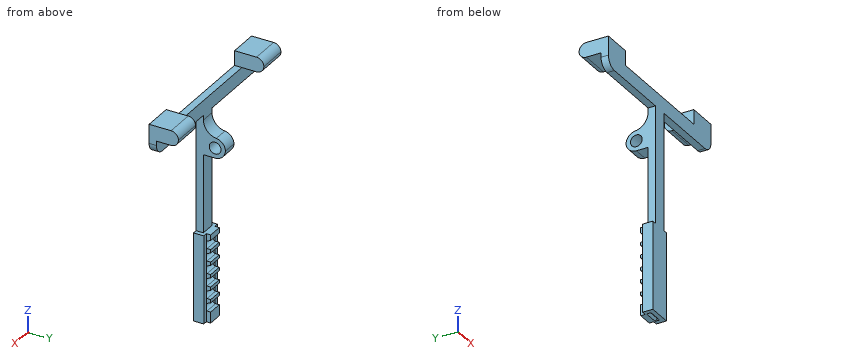
from build123d import *

# Parameters (mm, degrees)
BOSS_EXTRUDE1_DEPTH = 5
SKETCH1_3_W         = 20
SKETCH1_3_H         = 10
SKETCH1_3_W_2       = 10
SKETCH1_3_H_2       = 13.608990902
BOSS_EXTRUDE2_DEPTH = 20
SKETCH1_5_W         = 10
SKETCH1_5_H         = 60
BOSS_EXTRUDE3_DEPTH = 10
SKETCH3_R           = 4
CUT_EXTRUDE1_DEPTH  = 10
FILLET1_R           = 10
FILLET2_R           = 5
FILLET3_R           = 7
FILLET4_R           = 7
FILLET5_R           = 7
SKETCH1_6_W         = 3
SKETCH1_6_H         = 60
BOSS_EXTRUDE4_DEPTH = 7


# Some blends are built 0.0001 mm under size
with BuildPart() as part:
    # Sketch1 → Boss-Extrude1 (new body)
    with BuildSketch(Plane(origin=(0, 0, 0), x_dir=(1, 0, 0), z_dir=(0, 1, 0))):
        Polygon((40, -8.515763432), (40, -18.515763432), (60, -18.515763432), (60, 1.484236568), (5, 1.484236568), (5, 141.484236568), (-5, 141.484236568), (-5, 1.484236568), (-60, 1.484236568), (-60, -18.515763432), (-40, -18.515763432), (-40, -8.515763432), align=None)
    extrude(amount=BOSS_EXTRUDE1_DEPTH)

    # Sketch1<3> → Boss-Extrude2 (add)
    with BuildSketch(Plane(origin=(0, 0, 0), x_dir=(1, 0, 0), z_dir=(0, 1, 0))):
        with Locations((-50, -13.515763432)):
            Rectangle(SKETCH1_3_W, SKETCH1_3_H)
        Polygon((60, -8.515763432), (44.667493795, -8.515763432), (40, -8.515763432), (40, -18.515763432), (60, -18.515763432), align=None)
        with Locations((0, 21.484236568)):
            Rectangle(SKETCH1_3_W_2, SKETCH1_3_H_2)
    extrude(amount=BOSS_EXTRUDE2_DEPTH)

    # Sketch1<5> → Boss-Extrude3 (add)
    with BuildSketch(Plane(origin=(0, 0, 0), x_dir=(1, 0, 0), z_dir=(0, 1, 0))):
        with Locations((0, 111.484236568)):
            Rectangle(SKETCH1_5_W, SKETCH1_5_H)
    extrude(amount=BOSS_EXTRUDE3_DEPTH)

    # Sketch3 → Cut-Extrude1 (cut)
    with BuildSketch(Plane(origin=(5, 0, 0), x_dir=(0, 0, -1), z_dir=(1, 0, 0))):
        with Locations((21.484236568, 13)):
            Circle(SKETCH3_R)
        with BuildLine():
            Line((120.663634314, 6.570050981), (119.289130035, 10))
            Line((119.289130035, 10), (125.484236568, 10))
            Line((125.484236568, 10), (125.484236568, 7.5))
            ThreePointArc((125.484236568, 7.5), (123.457784012, 5.045259114), (120.663634314, 6.570050981))
        make_face()
        with BuildLine():
            Line((133.984236568, 7.5), (133.984236568, 10))
            Line((133.984236568, 10), (127.789130035, 10))
            Line((127.789130035, 10), (129.163634314, 6.570050981))
            ThreePointArc((129.163634314, 6.570050981), (131.957784012, 5.045259114), (133.984236568, 7.5))
        make_face()
        Polygon((141.484236568, 6), (139.984236568, 4.5), (141.484236568, 3), align=None)
        with BuildLine():
            Line((112.163634314, 6.570050981), (110.789130035, 10))
            Line((110.789130035, 10), (116.984236568, 10))
            Line((116.984236568, 10), (116.984236568, 7.5))
            ThreePointArc((116.984236568, 7.5), (114.957784012, 5.045259114), (112.163634314, 6.570050981))
        make_face()
        with BuildLine():
            Line((103.663634314, 6.570050981), (102.289130035, 10))
            Line((102.289130035, 10), (108.484236568, 10))
            Line((108.484236568, 10), (108.484236568, 7.5))
            ThreePointArc((108.484236568, 7.5), (106.457784012, 5.045259114), (103.663634314, 6.570050981))
        make_face()
        with BuildLine():
            Line((95.163634314, 6.570050981), (93.789130035, 10))
            Line((93.789130035, 10), (99.984236568, 10))
            Line((99.984236568, 10), (99.984236568, 7.5))
            ThreePointArc((99.984236568, 7.5), (97.957784012, 5.045259114), (95.163634314, 6.570050981))
        make_face()
        with BuildLine():
            Line((86.663634314, 6.570050981), (85.289130035, 10))
            Line((85.289130035, 10), (91.484236568, 10))
            Line((91.484236568, 10), (91.484236568, 7.5))
            ThreePointArc((91.484236568, 7.5), (89.457784012, 5.045259114), (86.663634314, 6.570050981))
        make_face()
    extrude(amount=-CUT_EXTRUDE1_DEPTH, mode=Mode.SUBTRACT)

    # Fillet1
    fillet1_edges = [part.edges().sort_by_distance(p)[0] for p in [
        (0, 5, -14.679741117),
    ]]
    fillet(fillet1_edges, radius=FILLET1_R)

    # Fillet2
    fillet2_edges = [part.edges().sort_by_distance(p)[0] for p in [
        (-50, 20, 8.515763432),
        (-50, 20, 18.515763432),
        (50, 20, 8.515763432),
        (50, 20, 18.515763432),
    ]]
    fillet(fillet2_edges, radius=FILLET2_R - 0.0001)  # a hair under: the kernel refuses the full size

    # Fillet3
    fillet3_edges = [part.edges().sort_by_distance(p)[0] for p in [
        (0, 20, -14.679741117),
    ]]
    fillet(fillet3_edges, radius=FILLET3_R)

    # Fillet4
    # the kernel refuses this fillet: 7 mm, written as the material it takes off along each edge
    with BuildSketch(Plane(origin=(22.486690858, 20, -28.288732019), x_dir=(0, 0, 1), z_dir=(-1, 0, 0))) as fillet4_piece_1:
        with BuildLine():
            CenterArc((7, -6.994676343), FILLET4_R, 92.234709992, 87.765290008)
            Line((0, -6.994676343), (-0.14, -6.994676343))
            Line((-0.14, -6.994676343), (-0.14, 0))
            Line((-0.14, 0), (0, 0.14))
            ThreePointArc((0, 0.14), (3.363523943, 0.14), (6.721588844, 0.139893527))
            Line((6.721588844, 0.139893527), (6.727047886, 0))
        make_face()
    extrude(amount=44.973381715, mode=Mode.SUBTRACT)

    # Fillet5
    fillet5_edges = [part.edges().sort_by_distance(p)[0] for p in [
        (-60, 2.5, -1.484236568),
        (60, 2.5, -1.484236568),
    ]]
    fillet(fillet5_edges, radius=FILLET5_R)

    # Sketch1<6> → Boss-Extrude4 (add)
    with BuildSketch(Plane(origin=(0, 0, 0), x_dir=(1, 0, 0), z_dir=(0, 1, 0))):
        with Locations((-6.5, 111.484236568)):
            Rectangle(SKETCH1_6_W, SKETCH1_6_H)
        with Locations((6.5, 111.484236568)):
            Rectangle(SKETCH1_6_W, SKETCH1_6_H)
    extrude(amount=BOSS_EXTRUDE4_DEPTH)


solid = part.part
Verification items for the finished model (mm, model axes). Coordinates: 2 decimals unless noted, no trailing zeros. Order: outer loops, then holes, each group sorted by start corner. A loop starts at its lowest first (then second) coordinate and runs counter-clockwise, first axis right, second up. Notation, with made-up numbers: M 0,68.5 L 50,68.5 A31 ccw 50,96.5 Z; hole C 67.25,34.25 d4. An arc over 180 degrees is marked long. One line per item, written item: value. Start each with the question number.
Item 1: Sectioned sample at B-B (z = -131). Enter the section's corners in (x, y).
Item 2: Gauge pin test, flat ends, axial feed: pin 1 (1.5 mm diameter, centred on y = 9, z = -83, fed in from +X); pin 2 (2.5 mm diameter, centred on x = 2, z = -110, fed in from +Y); pin 3 (2 mm diameter, centred on y = 6, z = -124, fed in from -X); pin 4 (6.5 mm diameter, centred on x = -2.5, y = 11, fed in from -Z). Record the tip position at first contact, or that the pin passes through.
Item 3: Sectioned sample at D-D (z = 3.5). Enter the section's corners in (x, y), then the cut area to 3 significant figures.
Item 4: Scan lines: probe 1 along X at (y, z) = (6.5, -87); probe 2 along Y at (x, z) = (2.5, -62.5); probe 3 along X at (y, z) = (7.5, -126.5). Record each from-to range of solid material in increasing order.
Item 5: Sectioned sample at C-C (z = -69.5). Enter the section's corners in (x, y).
Conclusion:
1. outline: M -8,0 L 8,0 L 8,7 L 5,7 L 5,5.05 L -5,5.05 L -5,7 L -8,7 Z
2. pin 1: stops at x = 5
2. pin 2: stops at y = 10
2. pin 3: stops at x = -8
2. pin 4: stops at z = -141.48
3. outline: M -59.7,0 L 59.7,0 L 59.7,5 L -59.7,5 Z
3. area: 597 mm^2
4. probe 1: x = -8 to -5, 5 to 8
4. probe 2: y = 0 to 5
4. probe 3: x = -5 to 5
5. outline: M -5,0 L 5,0 L 5,5 L -5,5 Z
